from build123d import *

# Parameters (mm, degrees)
SKETCH_1_W          = 25
SKETCH_1_H          = 15
SKETCH_1_W_2        = 22
SKETCH_1_H_2        = 12
EXTRUDE_1_DEPTH     = 150
SKETCH_2_R          = 1.6
SKETCH_2_R_2        = 9
CUT_EXTRUDE_1_DEPTH = 152.265495074


with BuildPart() as part:
    # ｽｹｯﾁ1 → ﾎﾞｽ - 押し出し1 (new body)
    with BuildSketch(Plane(origin=(0, 0, 0), x_dir=(1, 0, 0), z_dir=(0, 1, 0))):
        Rectangle(SKETCH_1_W, SKETCH_1_H)
        Rectangle(SKETCH_1_W_2, SKETCH_1_H_2, mode=Mode.SUBTRACT)
    extrude(amount=EXTRUDE_1_DEPTH)

    # ｽｹｯﾁ2 → ｶｯﾄ - 押し出し1 (cut, through all)
    with BuildSketch(Plane.XY.offset(7.5)):
        with Locations((5, 7.5)):
            Circle(SKETCH_2_R)
        with Locations((-5, 7.5)):
            Circle(SKETCH_2_R)
        with Locations(Location((5, 142.5, 0), (0, 0, 180))):
            Circle(SKETCH_2_R)
        with Locations(Location((-5, 142.5, 0), (0, 0, 180))):
            Circle(SKETCH_2_R)
        with Locations((0, 75)):
            Circle(SKETCH_2_R_2)
    extrude(amount=-CUT_EXTRUDE_1_DEPTH, mode=Mode.SUBTRACT)


solid = part.part
Part model, mm, in its own coordinate system. A direction names the side the tool comes from. Give positions to 0.01 mm unless a question says otherwise; leave off trailing zeros. Order: outer loops, then holes, each group sorted by start corner. A loop starts at its lowest first (then second) coordinate and runs counter-clockwise, first axis right, second up. Notation, with made-up numbers: (49.25, 78) -> (88.25, 78) arc R18 ccw to (88.25, 89) -> close; hole circle Ø1 at (66, -34.5). An arc over 180 degrees is marked (long way). Use one line per item in the form item = value.
(1) Saw through at A-A (z = 2.5). Write the cut outline in (x, y), then the cut area to 3 significant figures.
Solution:
outline = (-12.5, 0) -> (-11, 0) -> (-11, 150) -> (-12.5, 150) -> close; (11, 0) -> (12.5, 0) -> (12.5, 150) -> (11, 150) -> close
area = 450 mm²
(2) Tool access for faces 1 (the face through (-1.951, 66.214, -6.74)), 2 (the face through (-10, 74, -6)): list every direction of +Z, -Z, +X, -X, +Y, -Y with a clear straight run to the whole face (end or side of a thin tool).
Solution:
face_1 = +Z, -Z
face_2 = +Y, -Y
(3) Drill centre lines: line 1 (X direction, y = 124.5, z = 1.5); line 2 (Z direction, x = -2, y = 121); line 3 (Y direction, x = 0, z = 6.55). Where is each one in solid material? Low to high. Write a range as from..to.
Solution:
line_1 = -12.5..-11, 11..12.5
line_2 = -7.5..-6, 6..7.5
line_3 = 0..66, 84..150
(4) Pull direction Y, two halves, no side cores. Call faces 3 (the face through (-0.06, 150, -6.15)), 4 (the face through (5.35, 144.06, 6.76)), 5 (the face through (-11, 74, -7.5)): +Y half, -Y half, draft (parallel to the pull), parting line (faces both ways), or undercut.
Solution:
face_3 = +Y half
face_4 = undercut
face_5 = draft
(5) Saw through at C-C (y = 78). Write the cut outline in (x, z), then the cut area to 3 significant figures.
Solution:
outline = (-12.5, -7.5) -> (-8.49, -7.5) -> (-8.49, -6) -> (-11, -6) -> (-11, 6) -> (-8.49, 6) -> (-8.49, 7.5) -> (-12.5, 7.5) -> close; (8.49, -7.5) -> (12.5, -7.5) -> (12.5, 7.5) -> (8.49, 7.5) -> (8.49, 6) -> (11, 6) -> (11, -6) -> (8.49, -6) -> close
area = 60.1 mm²
(6) Saw through at B-B (y = 142.5). Write the cut outline in (x, z).
Solution:
outline = (-12.5, -7.5) -> (-6.6, -7.5) -> (-6.6, -6) -> (-11, -6) -> (-11, 6) -> (-6.6, 6) -> (-6.6, 7.5) -> (-12.5, 7.5) -> close; (-3.4, -7.5) -> (3.4, -7.5) -> (3.4, -6) -> (-3.4, -6) -> close; (-3.4, 6) -> (3.4, 6) -> (3.4, 7.5) -> (-3.4, 7.5) -> close; (6.6, -7.5) -> (12.5, -7.5) -> (12.5, 7.5) -> (6.6, 7.5) -> (6.6, 6) -> (11, 6) -> (11, -6) -> (6.6, -6) -> close
(7) Saw through at D-D (x = 5). Count the separate pieces of the cut face and the enclosed holes in it, then the cut area to 3 significant figures.
Solution:
separate_pieces = 8
enclosed_holes = 0
area = 386 mm²
(8) Flat gauge pin, fed straight in: P1, Ø5, axis at x = 2.5, z = -5, coming from the -Y side. Where does the tip first touch, or does it go through?
Solution:
P1 = 0
